from build123d import *

# Parameters (mm, degrees)
SKETCH1_W           = 220
SKETCH1_H           = 220
SKETCH1_R           = 85
SKETCH1_R_2         = 1.5
BOSS_EXTRUDE1_DEPTH = 24
CUT_EXTRUDE1_START  = -3
CUT_EXTRUDE1_DEPTH  = 3


with BuildPart() as part:
    # Sketch1 → Boss-Extrude1 (new body)
    with BuildSketch(Plane(origin=(0, 0, 0), x_dir=(1, 0, 0), z_dir=(0, 1, 0))):
        Rectangle(SKETCH1_W, SKETCH1_H)
        with Locations(Location((0, 0, 0), (0, 0, 270))):
            Circle(SKETCH1_R, mode=Mode.SUBTRACT)
        with Locations(Location((-105, 2.5, 0), (0, 0, 270))):
            Circle(SKETCH1_R_2, mode=Mode.SUBTRACT)
        with Locations(Location((-105, -2.5, 0), (0, 0, 270))):
            Circle(SKETCH1_R_2, mode=Mode.SUBTRACT)
        with Locations(Location((105, 2.5, 0), (0, 0, 270))):
            Circle(SKETCH1_R_2, mode=Mode.SUBTRACT)
        with Locations(Location((105, -2.5, 0), (0, 0, 270))):
            Circle(SKETCH1_R_2, mode=Mode.SUBTRACT)
        with Locations(Location((-2.5, -105, 0), (0, 0, 270))):
            Circle(SKETCH1_R_2, mode=Mode.SUBTRACT)
        with Locations(Location((2.5, -105, 0), (0, 0, 270))):
            Circle(SKETCH1_R_2, mode=Mode.SUBTRACT)
        with Locations(Location((-2.5, 105, 0), (0, 0, 270))):
            Circle(SKETCH1_R_2, mode=Mode.SUBTRACT)
        with Locations(Location((2.5, 105, 0), (0, 0, 270))):
            Circle(SKETCH1_R_2, mode=Mode.SUBTRACT)
    extrude(amount=BOSS_EXTRUDE1_DEPTH)

    # Sketch2 → Cut-Extrude1 (cut)
    with BuildSketch(Plane(origin=(0, 24, 0), x_dir=(1, 0, 0), z_dir=(0, 1, 0)).offset(CUT_EXTRUDE1_START)):
        with BuildLine():
            Line((4, 105), (4, -105))
            ThreePointArc((4, -105), (2.5, -106.5), (1, -105))
            Line((1, -105), (1, 105))
            ThreePointArc((1, 105), (2.5, 106.5), (4, 105))
        make_face()
        with BuildLine():
            Line((-1, 105), (-1, -105))
            ThreePointArc((-1, -105), (-2.5, -106.5), (-4, -105))
            Line((-4, -105), (-4, 105))
            ThreePointArc((-4, 105), (-2.5, 106.5), (-1, 105))
        make_face()
    extrude(amount=CUT_EXTRUDE1_DEPTH, mode=Mode.SUBTRACT)


solid = part.part
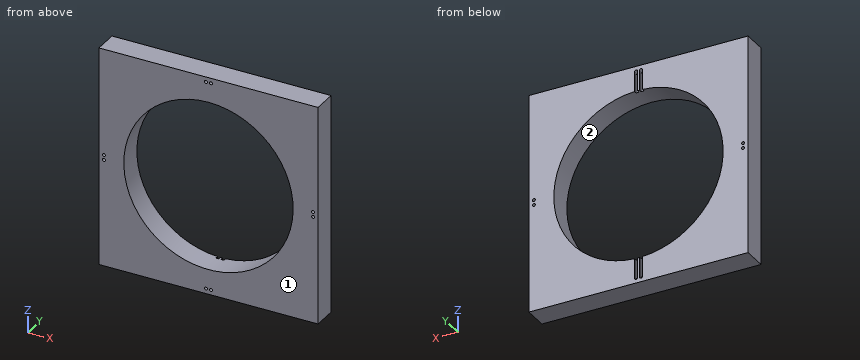
Part model, mm, in its own coordinate system. Face numbers are marked on the shaded views. Round coordinates to 2 decimals unless told otherwise and drop trailing zeros. Order: outer loops, then holes, each group sorted by start corner. A loop starts at its lowest first (then second) coordinate and runs counter-clockwise, first axis right, second up. Notation, with made-up numbers: (38, 4) -> (94, 4) arc R33 cw to (94, 37) -> close; hole circle Ø7 at (83, 84). An arc over 180 degrees is marked (long way). Put each result on its own line as item: value.
Q1. Band-saw the part on A-A (z = -75). Give the cut face in (x, y), and give its area (3 significant figures).
From the geometry:
outline: (-110, 0) -> (-40, 0) -> (-40, 24) -> (-110, 24) -> close; (40, 0) -> (110, 0) -> (110, 24) -> (40, 24) -> close
area: 3,360 mm2
Q2. Pull direction Z, two halves, no side cores. Call the marked faces 1 and 2: pulls with the +Z half, pulls with the -Z half, needs draft (parallel to the pull), parting line crosses it, or undercut.
From the geometry:
face 1: needs draft
face 2: undercut
Q3. Band-saw the part on B-B (y = 17). State how many separate pieces and enclosed holes the cut face has, and give its area (3 significant figures).
From the geometry:
separate pieces: 1
enclosed holes: 9
area: 25,600 mm2
Q4. Pin check, flat tips, straight feed: pin 1 Ø1.8 at (x, z) = (-2.5, -105) entering from +Y; pin 2 Ø2.5 at (x, z) = (-2.5, -99) entering from +Y. Stop position of each tip, or through.
From the geometry:
pin 1: passes through
pin 2: stops at y = 21
Q5. Wall check: line 1 (Z direction, x = -105, y = 17.5); line 2 (Z direction, x = -2.5, y = 19). Give the ranges that are in metal, low to high. Write a range as [from, to].
From the geometry:
line 1: z = [-110, -4], [-1, 1], [4, 110]
line 2: z = [-110, -106.5], [-103.5, -84.96], [84.96, 103.5], [106.5, 110]
Q6. Band-saw the part on C-C (x = -81.5). Give the cut face in (y, z), and give its area (3 significant figures).
From the geometry:
outline: (0, -110) -> (24, -110) -> (24, -24.14) -> (0, -24.14) -> close; (0, 24.14) -> (24, 24.14) -> (24, 110) -> (0, 110) -> close
area: 4,120 mm2
